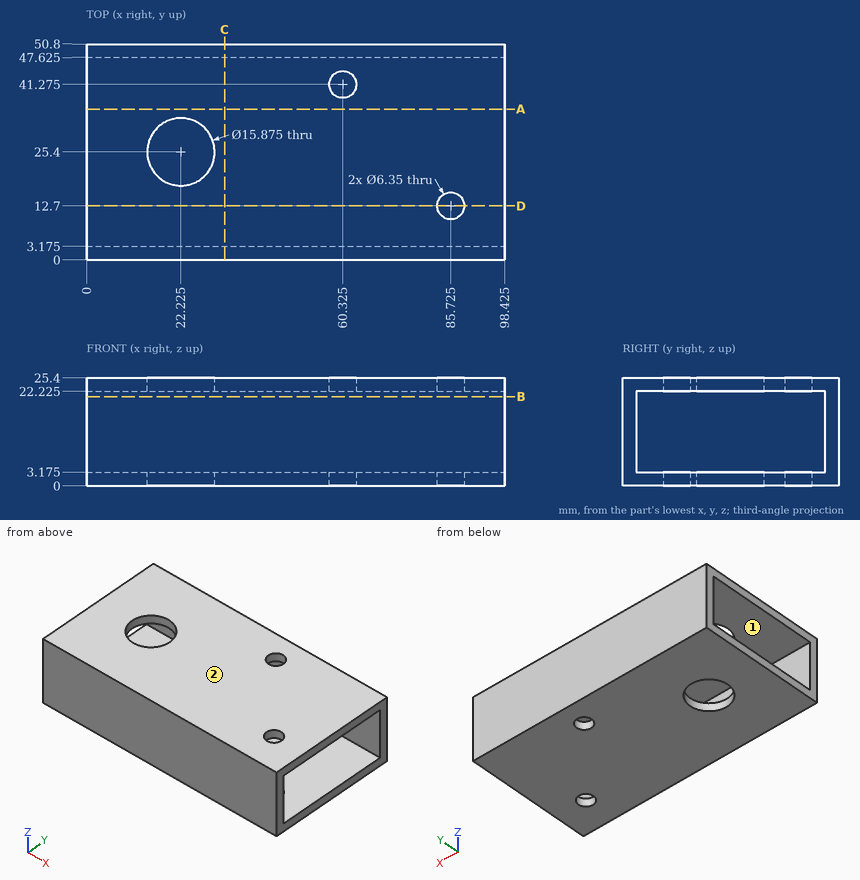
Can you work these out from the drawing? Everything is in mm from the part's minimum corner. A direction names the side the tool comes from. Coordinates: 2 decimals unless noted, no trailing zeros. Write each loop counter-clockwise with the first axis right and the second up, starting at its lowest first coordinate (ties: lowest second). Pieces come first, ordered by that corner, then holes. Notation, with made-up numbers: (4.5, 33.5) -> (11.5, 33.5) arc R18 cw to (11.5, 67.5) -> close; hole circle Ø11 at (-0.5, 35.5). An arc over 180 degrees is marked (long way). Write each question's results on one line, items separated by ' | '. Start each with the question number.
Q1. I'm going to push a flat-ended pin straight in: pin 1 (12.5 mm diameter, centred on x = 22.225, y = 25.4, fed in from -Z). Where does the tip first touch, or does it pass through?
Q2. Imagine slicing it at B-B (z = 21). Write out the boundary of the cut face in (x, y) (3 decimals), then the cut area to 3 significant figures.
Q3. Imagine slicing it at C-C (x = 32.5). Write out the boundary of the cut face in (y, z) (3 decimals).
Q4. On a 3-axis mill with a long thin cutter (end or side, diameter ignored), from which of +Z, -Z, +X, -X, +Y, -Y can I reach the whole of each face in a straight line? I mean the marked faces 1 and 2. Say none if no direction works.
Q5. If I drill on probe 1 along Y at (x, z) = (43.5, 16) (3 decimals); probe 2 along Z at (x, y) = (72, 4) (3 decimals); probe 3 along X at (y, z) = (25.4, 23.8) (1 decimal), over which ranges is the centre line in solid material (lowest first)?
Q6. Imagine slicing it at D-D (y = 12.7). Write out the boundary of the cut face in (x, z) (3 decimals).
Q7. Imagine slicing it at A-A (y = 35.5). Write out the boundary of the cut face in (x, z) (3 decimals).
Taken from the geometry:
1) pin 1: passes through
2) outline: (0, 0) -> (98.425, 0) -> (98.425, 3.175) -> (0, 3.175) -> close; (0, 47.625) -> (98.425, 47.625) -> (98.425, 50.8) -> (0, 50.8) -> close | area: 625 mm^2
3) outline: (0, 0) -> (50.8, 0) -> (50.8, 25.4) -> (0, 25.4) -> close; hole (3.175, 3.175) -> (47.625, 3.175) -> (47.625, 22.225) -> (3.175, 22.225) -> close
4) face 1: +X, -X | face 2: +Z, +X, -X, +Y, -Y
5) probe 1: y = 0 to 3.175, 47.625 to 50.8 | probe 2: z = 0 to 3.175, 22.225 to 25.4 | probe 3: x = 0 to 14.3, 30.2 to 98.4
6) outline: (0, 0) -> (82.55, 0) -> (82.55, 3.175) -> (0, 3.175) -> close; (0, 22.225) -> (82.55, 22.225) -> (82.55, 25.4) -> (0, 25.4) -> close; (88.9, 0) -> (98.425, 0) -> (98.425, 3.175) -> (88.9, 3.175) -> close; (88.9, 22.225) -> (98.425, 22.225) -> (98.425, 25.4) -> (88.9, 25.4) -> close
7) outline: (0, 0) -> (98.425, 0) -> (98.425, 3.175) -> (0, 3.175) -> close; (0, 22.225) -> (98.425, 22.225) -> (98.425, 25.4) -> (0, 25.4) -> close
